The figure shows three views and two pictorial views of one solid part (mm, origin at its lowest corner). Answer the questions. Round coordinates to 2 decimals unless told otherwise and drop trailing zeros. Write each loop counter-clockwise with the first axis right and the second up, starting at its lowest first coordinate (ties: lowest second). Pieces come first, ordered by that corner, then holes. Notation, with made-up numbers: M 26,-27 L 47,-27 A23 ccw 47,-5 Z; hole C 17,43 d2. An arc over 180 degrees is marked long. Answer in a Markdown table with one row per item.
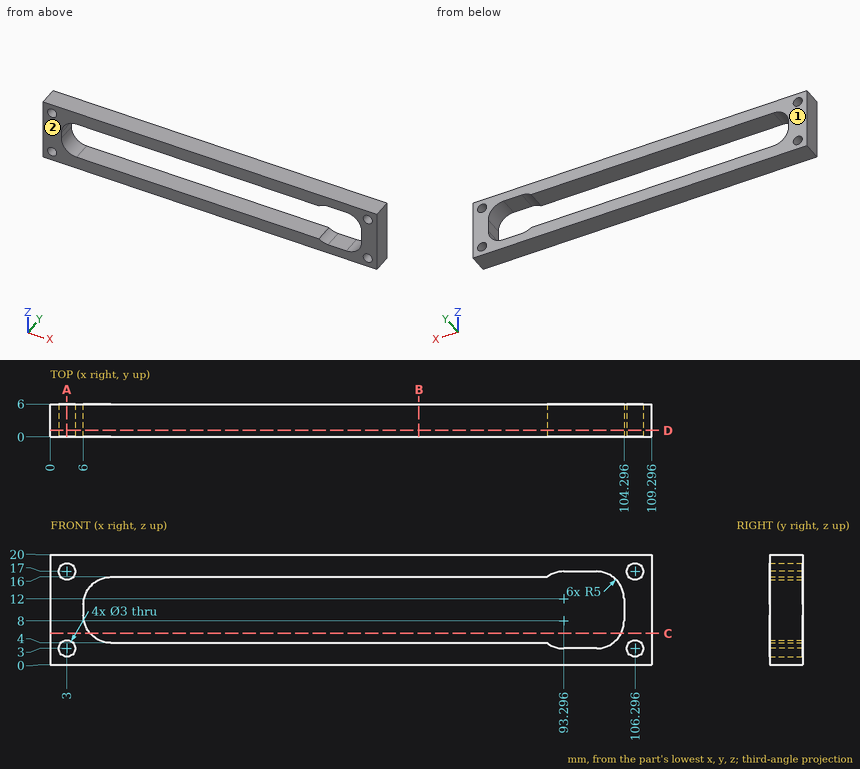
1. Given pin 1 (8 mm diameter, centred on x = 13, z = 8.5, fed in from +Y); pin 2 (3.5 mm diameter, centred on x = 3, z = 17, fed in from +Y), each flat-ended and moving along its own axis, determine where each tip first touches the part or whether it passes through.
Calculated:
| item | result |
|---|---|
| pin 1 | passes through |
| pin 2 | stops at y = 6 |
2. The part is cut by section B-B (x = 67). Determine the outline of the cut face in (y, z), plus the area to 3 significant figures.
Calculated:
| item | result |
|---|---|
| outline | M 0,0 L 6,0 L 6,4 L 0,4 Z; M 0,16 L 6,16 L 6,20 L 0,20 Z |
| area | 48.0 mm² |
3. Determine the mould class of the marked faces 1 and 2 for opening direction Y: released by +Y, released by -Y, zero draft, split by the parting line, or undercut.
Calculated:
| item | result |
|---|---|
| face 1 | released by +Y |
| face 2 | released by -Y |
4. The part is cut by section C-C (z = 5.75). Determine the outline of the cut face in (x, y), plus the area to 3 significant figures.
Calculated:
| item | result |
|---|---|
| outline | M 0,0 L 7.2,0 L 7.2,6 L 0,6 Z; M 103.76,0 L 109.3,0 L 109.3,6 L 103.76,6 Z |
| area | 76.4 mm² |
5. Consider line 1 along Z through (x, y) = (57, 0.55); line 2 along Z through (x, y) = (99, 5); line 3 along X through (y, z) = (3.85, 13.75). Determine where each line is inside the solid, lowest interval first. Write a range as from..to.
Calculated:
| item | result |
|---|---|
| line 1 | z = 0..4, 16..20 |
| line 2 | z = 0..3, 17..20 |
| line 3 | x = 0..6.82, 103.98..109.3 |
6. The part is cut by section A-A (x = 3). Determine the outline of the cut face in (y, z), plus the area to 3 significant figures.
Calculated:
| item | result |
|---|---|
| outline | M 0,0 L 6,0 L 6,1.5 L 0,1.5 Z; M 0,4.5 L 6,4.5 L 6,15.5 L 0,15.5 Z; M 0,18.5 L 6,18.5 L 6,20 L 0,20 Z |
| area | 84.0 mm² |
7. The part is cut by section D-D (y = 1.2). Determine the outline of the cut face in (x, z).
Calculated:
| item | result |
|---|---|
| outline | M 0,0 L 109.3,0 L 109.3,20 L 0,20 Z; hole C 3,3 d3; hole C 3,17 d3; hole M 6,9 A5 ccw 11,4 L 90.3,4 A5 ccw 93.3,3 L 99.3,3 A5 ccw 104.3,8 L 104.3,12 A5 ccw 99.3,17 L 93.3,17 A5 ccw 90.3,16 L 11,16 A5 ccw 6,11 Z; hole C 106.3,3 d3; hole C 106.3,17 d3 |
